Geometry check sheet. Reference: drawing and pictorial views, mm from the part's lowest x, y, z. Round coordinates to 2 decimals unless told otherwise and drop trailing zeros. Loops run counter-clockwise (first coordinate to the right, second up) from the corner with the lowest first, then second, coordinate; pieces in that order, holes last. Notation, with made-up numbers: (72, -4) - (107, -4) arc R16 cw to (107, 12) - close; hole circle Ø8 at (77, 9). An arc over 180 degrees is marked (long way). Answer as CSV lines item,"result". Start each with the question number.
1) Cross-section at A-A on x = 80. Record the boundary of the cut face in (y, z).
2) Depth check by flat-ended pin: P1, Ø0.9, axis at y = 1, z = 60, coming from the -X side; P2, Ø0.9, axis at x = 1, y = 1, coming from the +Z side; P3, Ø1.5, axis at x = 2, y = 1, coming from the -Z side. Enter the tip coordinate at first touch or a pass-through.
3) Thickness scan on line 1 along X through (y, z) = (1.55, 100.5). Record the ranges inside material, lowest first.
4) Cross-section at B-B on z = 56. Record the boundary of the cut face in (x, y), and give its area (3 significant figures).
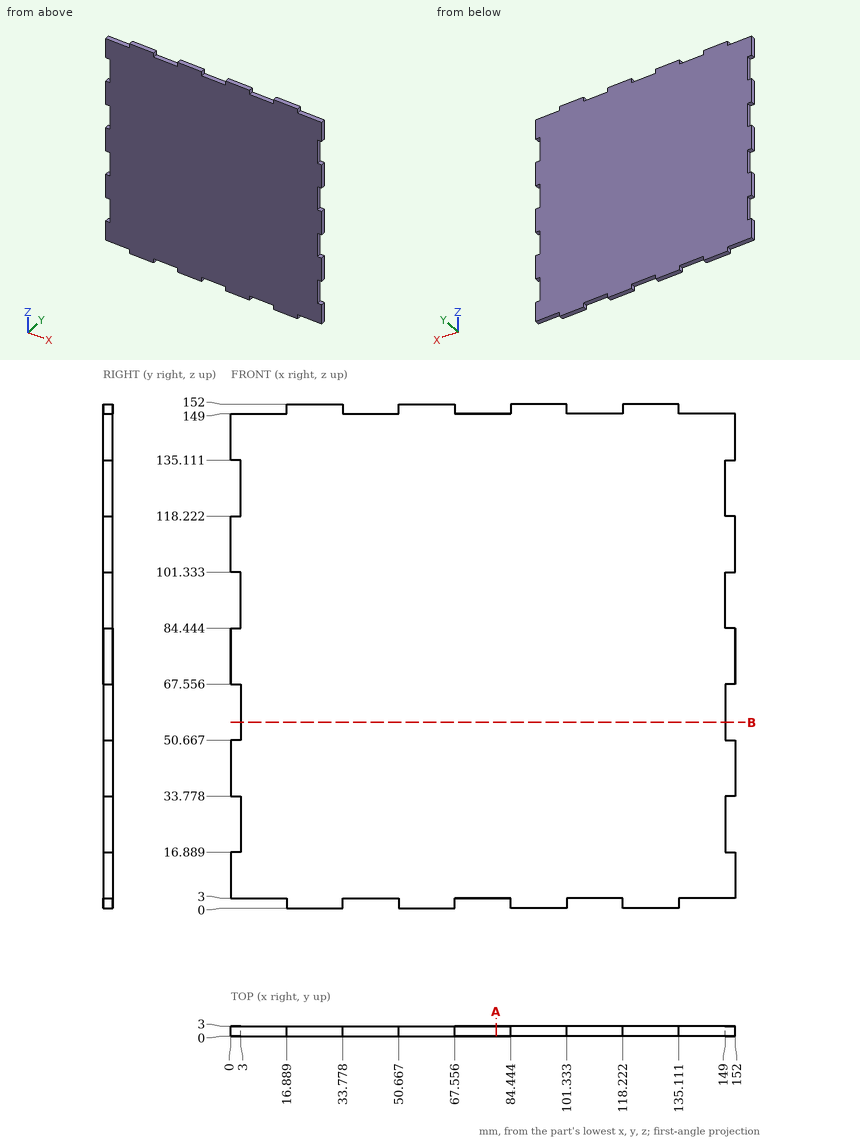
Answer block:
1,outline,"(0, 3) - (3, 3) - (3, 149) - (0, 149) - close"
2,P1,"stops at x = 3"
2,P2,"stops at z = 149"
2,P3,"stops at z = 3"
3,line 1,"x = 3 to 149"
4,outline,"(3, 0) - (149, 0) - (149, 3) - (3, 3) - close"
4,area,"438 mm^2"
